from build123d import *

# Parameters (mm, degrees)
SKETCH1_R           = 17.8
BOSS_EXTRUDE1_DEPTH = 20
SKETCH2_R           = 1.25
CUT_EXTRUDE1_DEPTH  = 12.7
CIRPATTERN1_COUNT   = 3
SKETCH3_R           = 1.5
CUT_EXTRUDE2_DEPTH  = 12.7
CIRPATTERN2_COUNT   = 4
CHAMFER1_SIZE       = 6
CUT_EXTRUDE3_START  = -8.382
SKETCH4_R           = 17.8
SKETCH4_R_2         = 2.5
CUT_EXTRUDE3_DEPTH  = 0.254


with BuildPart() as part:
    # Sketch1 → Boss-Extrude1 (new body, symmetric)
    with BuildSketch(Plane(origin=(0, 0, 0), x_dir=(1, 0, 0), z_dir=(0, 1, 0))):
        Circle(SKETCH1_R)
    extrude(amount=BOSS_EXTRUDE1_DEPTH, both=True)

    # Sketch2 → Cut-Extrude1 (cut)
    with BuildSketch(Plane(origin=(0, 20, 0), x_dir=(1, 0, 0), z_dir=(0, 1, 0))):
        with Locations((0, 6.5)):
            Circle(SKETCH2_R)
    cut_extrude1 = extrude(amount=-CUT_EXTRUDE1_DEPTH, mode=Mode.SUBTRACT)

    # CirPattern1: Cut-Extrude1 ×3 about axis
    cirpattern1_axis = Axis((0, 0, 0), (0, 1, 0))
    for i in range(1, CIRPATTERN1_COUNT):
        add(cut_extrude1.rotate(cirpattern1_axis, i * 360 / CIRPATTERN1_COUNT), mode=Mode.SUBTRACT)

    # Sketch3 → Cut-Extrude2 (cut)
    with BuildSketch(Plane.XZ.offset(20)):
        with Locations((0, 12.5)):
            Circle(SKETCH3_R)
    cut_extrude2 = extrude(amount=-CUT_EXTRUDE2_DEPTH, mode=Mode.SUBTRACT)

    # CirPattern2: Cut-Extrude2 ×4 about axis
    cirpattern2_axis = Axis((0, 0, 0), (0, 1, 0))
    for i in range(1, CIRPATTERN2_COUNT):
        add(cut_extrude2.rotate(cirpattern2_axis, i * 360 / CIRPATTERN2_COUNT), mode=Mode.SUBTRACT)

    # Chamfer1
    chamfer1_edges = [part.edges().sort_by_distance(p)[0] for p in [
        (-17.8, 20, 0),
    ]]
    chamfer(chamfer1_edges, length=CHAMFER1_SIZE)

    # Sketch4 → Cut-Extrude3 (cut)
    with BuildSketch(Plane.XZ.offset(20).offset(CUT_EXTRUDE3_START)):
        Circle(SKETCH4_R)
        Circle(SKETCH4_R_2, mode=Mode.SUBTRACT)
    extrude(amount=-CUT_EXTRUDE3_DEPTH, mode=Mode.SUBTRACT)


solid = part.part
Read the model definition and answer for the solid it produces. Units are mm, in the model's axes. A direction names the side the tool comes from. Coordinates: 2 decimals unless noted, no trailing zeros. Write each loop counter-clockwise with the first axis right and the second up, starting at its lowest first coordinate (ties: lowest second). Pieces come first, ordered by that corner, then holes. Notation, with made-up numbers: M 20,-28.5 L 37,-28.5 A15 ccw 37,-8.5 Z; hole C 66.25,8.25 d9. An arc over 180 degrees is marked long. Use a Markdown table: item, result.
Q1. The part is cut by section A-A, the plane x = 0. Give the number of separate pieces and of enclosed holes in the cut face, then the cut area to 3 significant figures.
Answer block:
| item | result |
|---|---|
| separate pieces | 3 |
| enclosed holes | 0 |
| area | 1,270 mm2 |
Q2. Straight lines are drawn through the part: L1, parallel to Y at x = -2, z = -5; L2, parallel to X at y = -14, z = 0. For each, find the intervals that lie inside material, in ascending order. Write a range as [from, to].
Answer block:
| item | result |
|---|---|
| L1 | y = [-20, -11.62], [-11.36, 20] |
| L2 | x = [-17.8, -14], [-11, 11], [14, 17.8] |
Q3. Which of the six approach directions +Z, -Z, +X, -X, +Y, -Y give full straight-line access (tool end or side, diameter ignored) to faces 5 (the face through (-11, -16, 0)), 6 (the face through (0, 20, 0)), 7 (the face through (-6, 7.3, 3))?
Answer block:
| item | result |
|---|---|
| face 5 | -Y |
| face 6 | +Z, -Z, +X, -X, +Y |
| face 7 | +Y |
Q4. Determine the mould class of faces 1 (the face through (0, -7.3, 13)), 2 (the face through (0, -11.364, -4)), 3 (the face through (4.38, 13.74, 3.2)), 4 (the face through (-12.08, 19.71, -0.53)) for opening direction Z: released by +Z, released by -Z, zero draft, split by the parting line, or undercut.
Answer block:
| item | result |
|---|---|
| face 1 | undercut |
| face 2 | zero draft |
| face 3 | undercut |
| face 4 | split by the parting line |
Q5. The part is cut by section D-D, the plane y = 9.5. Write down the section's boundary in (x, z).
Answer block:
| item | result |
|---|---|
| outline | C 0,0 d35.6; hole C -5.63,3.25 d2.5; hole C 0,-6.5 d2.5; hole C 5.63,3.25 d2.5 |
Q6. The part is cut by section C-C, the plane y = -8. Write down the section's boundary in (x, z), then the cut area to 3 significant figures.
Answer block:
| item | result |
|---|---|
| outline | C 0,0 d35.6; hole C -12.5,0 d3; hole C 0,-12.5 d3; hole C 0,12.5 d3; hole C 12.5,0 d3 |
| area | 967 mm2 |
Q7. Each of these flat-tipped pins is pushed along its axis until it touches: pin 1 Ø2.5 at (x, z) = (-12.5, 0) entering from -Y; pin 2 Ø2 at (x, y) = (8, -5.5) entering from -Z; pin 3 Ø5 at (y, z) = (-15.5, 9) entering from +X. Where does it stop, or does it pass through?
Answer block:
| item | result |
|---|---|
| pin 1 | stops at y = -7.3 |
| pin 2 | stops at z = -16.37 |
| pin 3 | stops at x = 16.57 |
